```python
from build123d import *

# Parameters (mm, degrees)
SKETCH1_R           = 1.750000093
SKETCH1_R_2         = 1.749998765
BOSS_EXTRUDE1_DEPTH = 4.00000019


with BuildPart() as part:
    # Sketch1 → Boss-Extrude1 (new body)
    with BuildSketch(Plane(origin=(0, 4.00000019, 0), x_dir=(1, 0, 0), z_dir=(0, 1, 0))):
        Polygon((32.525639981, -7.142858114), (32.88276121, -7.393712178), (33.265069127, -7.604169194), (33.66804868, -7.771722972), (34.086868167, -7.894380018), (34.516561776, -7.97067862), (34.952010959, -7.99971167), (35.388030112, -7.981133647), (35.81944108, -7.915167138), (36.241080612, -7.802593987), (36.647960544, -7.644756231), (37.035208195, -7.443531882), (37.39824146, -7.201318163), (37.732720375, -6.920996122), (38.034681231, -6.605904084), (38.300510496, -6.259791087), (38.527049124, -5.886779167), (38.711611181, -5.491307005), (38.85198012, -5.078083836), (38.946498185, -4.652027041), (38.994051516, -4.218208138), (38.994051516, -3.781792009), (38.946498185, -3.347974038), (38.85198012, -2.92191701), (38.711611181, -2.508692909), (38.527049124, -2.11322098), (38.300510496, -1.740208943), (38.034681231, -1.394096995), (37.732720375, -1.079004025), (37.39824146, -0.798682508), (37.035208195, -0.556467974), (36.647960544, -0.355244207), (36.241080612, -0.197406596), (35.81944108, -0.084833708), (35.388030112, -0.0188658), (34.952010959, -0.000288244), (34.516561776, -0.02932176), (34.086868167, -0.105620798), (33.66804868, -0.228277393), (33.265069127, -0.39583139), (32.88276121, -0.606288377), (32.525639981, -0.857143023), (32.252710313, -1.048453967), (31.960248947, -1.208308968), (31.65185824, -1.334734028), (31.331341714, -1.42616895), (31.002659351, -1.481484971), (30.669869855, -1.500000013), (8.330127224, -1.500000013), (7.997341454, -1.481484971), (7.668660954, -1.42616895), (7.348147221, -1.334734028), (7.039752789, -1.208308968), (6.747287232, -1.048453967), (6.474358961, -0.857143023), (6.117243785, -0.606288377), (5.73492609, -0.39583139), (5.331956781, -0.228277393), (4.913132172, -0.105620798), (4.483437166, -0.02932176), (4.047987983, -0.000288244), (3.611967899, -0.0188658), (3.180566011, -0.084833708), (2.758919029, -0.197406596), (2.352046082, -0.355244207), (1.964788884, -0.556467974), (1.601757947, -0.798682508), (1.267276006, -1.079004025), (0.965322892, -1.394096995), (0.699493627, -1.740208943), (0.472952612, -2.11322098), (0.288396404, -2.508692909), (0.148022096, -2.92191701), (0.053500291, -3.347974038), (0.005956274, -3.781792009), (0.005956274, -4.218208138), (0.053500291, -4.652027041), (0.148022096, -5.078083836), (0.288396404, -5.491307005), (0.472952612, -5.886779167), (0.699493627, -6.259791087), (0.965322892, -6.605904084), (1.267276006, -6.920996122), (1.601757947, -7.201318163), (1.964788884, -7.443531882), (2.352046082, -7.644756231), (2.758919029, -7.802593987), (3.180566011, -7.915167138), (3.611967899, -7.981133647), (4.047987983, -7.99971167), (4.483437166, -7.97067862), (4.913132172, -7.894380018), (5.331956781, -7.771722972), (5.73492609, -7.604169194), (6.117243785, -7.393712178), (6.474358961, -7.142858114), (6.747287232, -6.951545831), (7.039752789, -6.791692227), (7.348147221, -6.66526705), (7.668660954, -6.573832128), (7.997341454, -6.518514827), (8.330127224, -6.500000134), (30.669869855, -6.500000134), (31.002659351, -6.518514827), (31.331341714, -6.573832128), (31.65185824, -6.66526705), (31.960248947, -6.791692227), (32.252710313, -6.951545831), align=None)
        with Locations((4.006235525, -3.998948436)):
            Circle(SKETCH1_R, mode=Mode.SUBTRACT)
        with Locations((35.000000078, -3.999998668)):
            Circle(SKETCH1_R_2, mode=Mode.SUBTRACT)
    extrude(amount=-BOSS_EXTRUDE1_DEPTH)


solid = part.part
```
Here's how the part is built. I have some questions about the finished solid (model axes, mm). A direction names the side the tool comes from. Round coordinates to 2 decimals unless told otherwise and drop trailing zeros. Order: outer loops, then holes, each group sorted by start corner. A loop starts at its lowest first (then second) coordinate and runs counter-clockwise, first axis right, second up. Notation, with made-up numbers: M 71.25,-38 L 85.25,-38 A28 ccw 85.25,1 Z; hole C -22.75,-23.75 d5. An arc over 180 degrees is marked long. Answer as CSV lines item,"result".
Item 1: We'd pull the mould along X, two halves only. Please class faces 1 (the flat face through (19, 2, 6.5)), 2 (the flat face through (19, 4, 4)): +X half, -X half, draft (parallel to the pull), parting line (faces both ways), or undercut.
From the geometry:
face 1,"undercut"
face 2,"draft"
Item 2: Which directions (+Z, -Z, +X, -X, +Y, -Y) give clear straight access to the entire face, cutting with the end or side of a thin tool? Please do faces 3 (the cylindrical face through (3.6, 2, 5.7)), 4 (the flat face through (20, 2, 1.5)).
From the geometry:
face 3,"+Y, -Y"
face 4,"-Z, +Y, -Y"
Item 3: Imagine slicing it at B-B on x = 24. List the corners of the cut face in (y, z) for me.
From the geometry:
outline,"M 0,1.5 L 4,1.5 L 4,6.5 L 0,6.5 Z"
Item 4: For pin 1 (2 mm diameter, centred on x = 35, z = 4, fed in from +Y); pin 2 (2 mm diameter, centred on x = 25, y = 2, fed in from -Z), each with a flat end and sliding along its axis, tell me the tip position at first contact or that it passes through.
From the geometry:
pin 1,"through"
pin 2,"z = 1.5"
Item 5: Imagine slicing it at A-A on y = 3.15. Give the number of separate pieces and of enclosed holes in the cut face, and give its area (3 significant figures).
From the geometry:
separate pieces,"1"
enclosed holes,"2"
area,"200 mm2"
Item 6: Please list where these lines run through material, in increasing order: L1, parallel to X at y = 0.9, z = 4; L2, parallel to Z at x = 35, y = 3.7; L3, parallel to X at y = 1.85, z = 3. Write a range as [from, to].
From the geometry:
L1,"[0.01, 2.26], [5.76, 33.25], [36.75, 38.99]"
L2,"[0, 2.25], [5.75, 8]"
L3,"[0.13, 2.57], [5.44, 33.56], [36.44, 38.87]"
